The model under review builds one solid part; all positions refer to its coordinate system, in mm. Face numbers are marked on the shaded views. A direction names the side the tool comes from. Give positions to 0.01 mm unless a question says otherwise; leave off trailing zeros. Loops run counter-clockwise (first coordinate to the right, second up) from the corner with the lowest first, then second, coordinate; pieces in that order, holes last. Notation, with made-up numbers: M 41,48.5 L 63,48.5 A11 cw 63,58.5 Z; hole C -6.5,68.5 d11. An arc over 180 degrees is marked long. One line per item, written item: value. Start each with the question number.
Q1. For the marked faces 4 and 5, list the 3-axis set-ups (+Z, -Z, +X, -X, +Y, -Y) from which the entire face can be reached by the end or side of a thin tool; tool diameter is ignored.
Q2. We need section C-C on z = -7. Write out the cut boundary in (x, y).
Q3. We need section A-A on y = 5.5. Write out the cut boundary in (x, z), plus the area to 3 significant figures.
Q4. Mouldability with a two-part tool opening along Z and no side actions: class the marked faces 1, 2 and 3 as released by +Z, released by -Z, zero draft, split by the parting line, or undercut.
Q5. We need section D-D on y = 1. Write out the cut boundary in (x, z), plus the area to 3 significant figures.
Q6. To check wall thickness, follow line 1 along Z through (x, y) = (0, 5.25); line 2 along Z through (x, y) = (0, 1.75); line 3 along X through (y, z) = (0.5, 0). State the ranges of each line that lie inside material, in increasing order. Write a range as from..to.
Q7. For pin 1 (3.5 mm diameter, centred on x = 0, z = 0, fed in from +Y); pin 2 (6 mm diameter, centred on x = 2, z = 7, fed in from +Y); pin 3 (3 mm diameter, centred on x = -1.5, z = 0.5, fed in from +Y); pin 4 (5 mm diameter, centred on x = 0, z = 0, fed in from +Y), all flat-tipped, find the tip position at first contact; note any pin that passes through.
Autodesk Inventor part; units mm, degrees
ref_plane "YZ Plane" through (0, 0, 0) normal (1, 0, 0) x (0, 1, 0)
ref_plane "XZ Plane" through (0, 0, 0) normal (0, 1, 0) x (-1, 0, 0)
ref_plane "XY Plane" through (0, 0, 0) normal (0, 0, 1) x (1, 0, 0)
sketch "Sketch1" plane through (0, 0, 0) normal (0, 1, 0) x (-1, 0, 0)
  line L0 (5, 18) -> (-5, 18)
  line L1 (-5, 18) -> (-5, -18)
  line L2 (-5, -18) -> (5, -18)
  line L3 (5, -18) -> (5, 18)
  line L4 (5, 18) -> (-5, -18) construction
  line L5 (-5, 18) -> (5, -18) construction
  line L6 (5, -18) -> (5, -11)
  line L7 (5, -11) -> (-5, -11)
  point P0 (0, 0)
  dimension "d0" = 10
  dimension "d1" = 36
  dimension "d2" = 7
extrude "Extrusion1" add sketch "Sketch1" along normal blind 13 contours L3 L7 L1 L0
extrude "Extrusion2" add sketch "Sketch1" along normal blind 15 contours L3 L2 L1 L7
fillet "Fillet1" radius 2 4 edges at (0, 15, -11) (0, 13, -11) (0, 15, -18) (0, 13, 18)
sketch "Sketch2" plane through (0, 13, 0) normal (0, 1, 0) x (1, 0, 0)
  circle A0 centre (0, 0) radius 4
  circle A1 centre (0, 0) radius 2
  dimension "d8" = 8
  dimension "d9" = 4
extrude "Extrusion3" cut sketch "Sketch2" against normal blind 15 contours A1
extrude "Extrusion4" cut sketch "Sketch2" against normal blind 10
fillet "Fillet2" radius 1 2 edges at (-2, 3, 0) (-4, 13, 0)
properties part number "offset_vacuumbox"
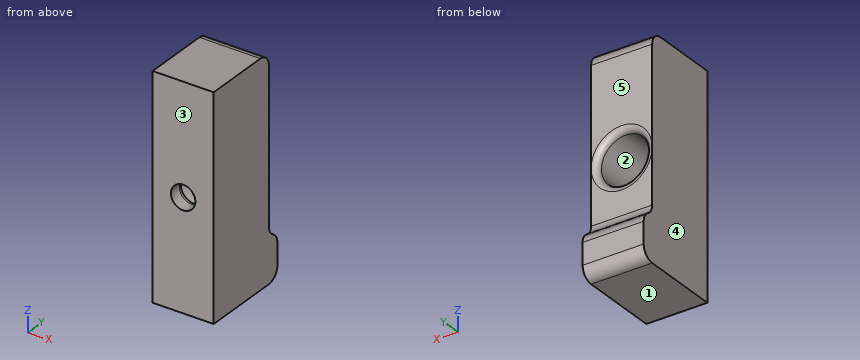
Solved:
1. face 4: +Z, -Z, -X, +Y, -Y
1. face 5: +Z, +X, -X, +Y
2. outline: M -5,0 L 5,0 L 5,13 L -5,13 Z
3. outline: M -5,-18 L 5,-18 L 5,18 L -5,18 Z; hole C 0,0 d8
3. area: 310 mm2
4. face 1: released by -Z
4. face 2: undercut
4. face 3: zero draft
5. outline: M -5,-18 L 5,-18 L 5,18 L -5,18 Z; hole C 0,0 d4
5. area: 347 mm2
6. line 1: -18..-4, 4..18
6. line 2: -18..-2, 2..18
6. line 3: -5..-2, 2..5
7. pin 1: through
7. pin 2: y = 13
7. pin 3: y = 3
7. pin 4: y = 2.87
